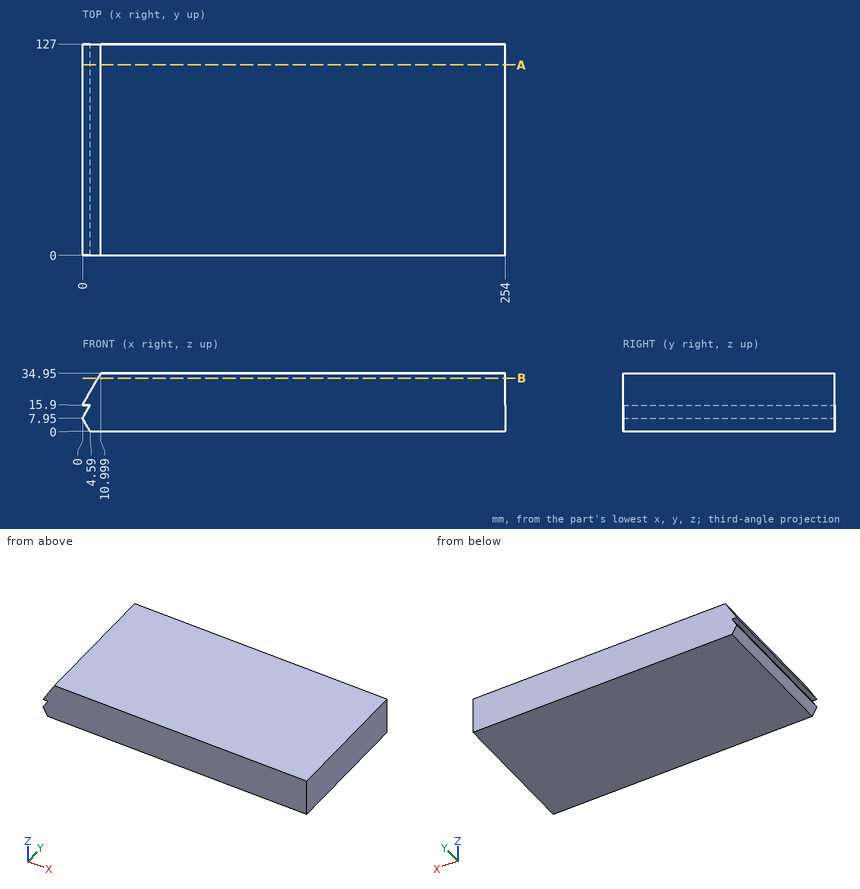
Check sheet for the drawn part. Datum: minimum x, y, z corner. Units: mm. Coordinates: 2 decimals unless noted, no trailing zeros. Write each loop counter-clockwise with the first axis right and the second up, starting at its lowest first coordinate (ties: lowest second). Pieces come first, ordered by that corner, then holes. Notation, with made-up numbers: M 20.5,57.5 L 29.5,57.5 A31 ccw 29.5,86.5 Z; hole C -20,35.5 d10. An arc over 180 degrees is marked long. Use a Markdown table: item, result.
Q1. Sectioned sample at B-B, the plane z = 32. Record the boundary of the cut face in (x, y) (1 decimal), plus the area to 3 significant figures.
Reply:
| item | result |
|---|---|
| outline | M 9.3,0 L 254,0 L 254,127 L 9.3,127 Z |
| area | 31,100 mm² |
Q2. Sectioned sample at A-A, the plane y = 114.5. Record the boundary of the cut face in (x, z).
Reply:
| item | result |
|---|---|
| outline | M 0,7.95 L 4.59,0 L 254,0 L 254,34.95 L 11,34.95 L 0,15.9 L 4.59,15.9 Z |
Q3. Go/stop test with flat-tipped pins: P1, Ø2, axis at y = 66, z = 5.5, coming from the -X side; P2, Ø1.4, axis at x = 3, y = 38, coming from the -Z side. Record where each tip stops, or that it passes through.
Reply:
| item | result |
|---|---|
| P1 | stops at x = 0.84 |
| P2 | stops at z = 1.54 |
Q4. Thickness scan on line 1 (X direction, y = 63, z = 16); line 2 (X direction, y = 104.5, z = 29.5). Record the ranges inside material, lowest first.
Reply:
| item | result |
|---|---|
| line 1 | x = 0.06 to 254 |
| line 2 | x = 7.85 to 254 |
